```python
from build123d import *

# Parameters (mm, degrees)
F0_W     = 5
F0_H     = 5
F1_DEPTH = 14
F2_DEPTH = 9
F3_R     = 3.5
F3_R_2   = 0.5
F4_DEPTH = 9
F5_R     = 0.55


with BuildPart() as f1:
    # F0 (on Top) → F1 (new body)
    with BuildSketch(Plane.XY):
        Rectangle(F0_W, F0_H)
    extrude(amount=F1_DEPTH)

    # F0 (on Top) → F2 (join)
    with BuildSketch(Plane.XY):
        Polygon((-2.5, 2.5), (2.5, 2.5), (2.5, 4.5), (-2.5, 4.9594354583), align=None)
        Polygon((2.5, -4.5), (2.5, -2.5), (-2.5, -2.5), (-2.5, -4.9594354583), align=None)
    extrude(amount=F2_DEPTH)

    # F3 (on face) → F4 (join)
    with BuildSketch(Plane.YZ.offset(2.5)):
        with Locations((0, 4)):
            Circle(F3_R)
        with Locations((0, 4)):
            Circle(F3_R_2, mode=Mode.SUBTRACT)
    extrude(amount=F4_DEPTH)

    # F5
    f5_edges = [f1.edges().sort_by_distance(p)[0] for p in [
        (2.5, -3.5, 4),
        (11.5, -3.5, 4),
    ]]
    fillet(f5_edges, radius=F5_R)


solid = f1.part
```
Geometry: final body of the model. Coordinates: model frame, mm. A direction names the side the tool comes from. Coordinates: 2 decimals unless noted, no trailing zeros. Order: outer loops, then holes, each group sorted by start corner. A loop starts at its lowest first (then second) coordinate and runs counter-clockwise, first axis right, second up. Notation, with made-up numbers: (71, -15.75) - (107, -15.75) arc R28 ccw to (107, 7.25) - close; hole circle Ø10 at (79, 2). An arc over 180 degrees is marked (long way). Return JSON: item names as keys, results as strings. Group by question number.
1. Cut plane C-C (x = 4.75). Output: boundary loops of the cut face in (y, z), plus the area to 3 significant figures.
2. Pin query (flat end, axial travel): pin 1 (2.5 mm diameter, centred on x = 1, z = 11.5, fed in from -Y); pin 2 (0.5 mm diameter, centred on y = 0, z = 4, fed in from +X); pin 3 (2 mm diameter, centred on x = 9.5, y = -1.5, fed in from -Z). Return the tip coordinate at first contact, or that it passes through.
3. Material intervals for line 1 along Z through (x, y) = (7.5, 0); line 2 along X through (y, z) = (3, 8); line 3 along Z through (x, y) = (0.5, -3.25), sorted ascending. Write a range as [from, to].
4. Pull-direction query (Y, two-part tool) for faces 1 (the face through (6.937, -0.065, 4.496)), 2 (the face through (2.5, -0.1, 8.5)), 3 (the face through (0, -2.5, 11)); classes: pulls with the +Y half, pulls with the -Y half, needs draft (parallel to the pull), parting line crosses it, or undercut.
5. Set-up query: faces 4 (the face through (0, -4, 9)), 5 (the face through (0, 0, 0)), 6 (the face through (-0.035, -4.733, 4.437)), 7 (the face through (0, 4, 9)), 8 (the face through (6.943, -0.759, 0.583)). Return all of +Z, -Z, +X, -X, +Y, -Y with unobstructed straight access to the full face (end or side cutting, diameter ignored); none if empty.
6. Cut plane B-B (x = -1). Output: boundary loops of the cut face in (y, z).
7. Cut plane D-D (z = 12). Output: boundary loops of the cut face in (x, y), plus the area to 3 significant figures.
8. Cut plane A-A (z = 4). Output: boundary loops of the cut face in (x, y).
Resolved:
{
 "1": {"outline": "circle Ø7 at (0, 4); hole circle Ø1 at (0, 4)", "area": "37.7 mm²"},
 "2": {"pin 1": "stops at y = -2.5", "pin 2": "stops at x = 2.5", "pin 3": "stops at z = 0.54"},
 "3": {"line 1": "z = [0.5, 3.5], [4.5, 7.5]", "line 2": "x = [-2.5, 2.5]", "line 3": "z = [0, 9]"},
 "4": {"face 1": "undercut", "face 2": "needs draft", "face 3": "pulls with the -Y half"},
 "5": {"face 4": "+Z, +X, -X, -Y", "face 5": "-Z, +X, -X, +Y, -Y", "face 6": "+Z, -Z, +X, -Y", "face 7": "+Z, +X, -X, +Y", "face 8": "+X"},
 "6": {"outline": "(-4.82, 0) - (4.82, 0) - (4.82, 9) - (2.5, 9) - (2.5, 14) - (-2.5, 14) - (-2.5, 9) - (-4.82, 9) - close"},
 "7": {"outline": "(-2.5, -2.5) - (2.5, -2.5) - (2.5, 2.5) - (-2.5, 2.5) - close", "area": "25.0 mm²"},
 "8": {"outline": "(-2.5, -4.96) - (2.5, -4.5) - (2.5, -4.05) arc R0.55 cw to (3.05, -3.5) - (10.95, -3.5) arc R0.55 ccw to (11.5, -2.95) - (11.5, -0.5) - (2.5, -0.5) - (2.5, 0.5) - (11.5, 0.5) - (11.5, 2.95) arc R0.55 ccw to (10.95, 3.5) - (3.05, 3.5) arc R0.55 cw to (2.5, 4.05) - (2.5, 4.5) - (-2.5, 4.96) - close"}
}
